Build history of the part. All positions in model axes, mm. A direction names the side the tool comes from. Round coordinates to 2 decimals unless told otherwise and drop trailing zeros. Write each loop counter-clockwise with the first axis right and the second up, starting at its lowest first coordinate (ties: lowest second). Pieces come first, ordered by that corner, then holes.
1) Pull direction X, two halves, no side cores. Call faces 6 (the flat face through (-145.011, 25, -16)), 7 (the cylindrical face through (-150.961, -14.765, -3.279)), 8 (the flat face through (-163.99, 16, -8)), 9 (the cylindrical face through (-146.66, -8.77, 27.84)): +X half, -X half, draft (parallel to the pull), parting line (faces both ways), or undercut.
2) Saw through at A-A (x = -81.5). Write the cut outline in (y, z), plus the area to 3 significant figures.
3) Which spindle directions (+Z, -Z, +X, -X, +Y, -Y) get a long thin tool onto all of the face, cutting with end or side? Do faces 1 (the flat face through (-90, -11.867, 0)), 2 (the conical face through (-144.014, -12.426, 39.459)), 3 (the flat face through (-122.028, 38, 92)), 4 (the cylindrical face through (-163.5, -4.84, 15.38)), 5 (the flat face through (-43.19, 7, 7)). Say none if no direction does.
4) Wall check: probe 1 along Y at (x, z) = (-163.45, 0) (3 decimals); probe 2 along Y at (x, z) = (-148, 0) (3 decimals); probe 3 along X at (y, z) = (57.5, -5). Give the ranges that are in metal, low to high.
5) Flat gauge pins, fed straight in: pin 1 (12 mm diameter, centred on x = -113, z = -47, fed in from -Y); pin 2 (2.5 mm diameter, centred on x = -74.5, z = -1, fed in from +Y); pin 3 (1.5 mm diameter, centred on x = -72.5, z = -21.5, fed in from +Y); pin 4 (24 mm diameter, centred on y = 0, z = 0, fed in from +X). Where does each tip first touch, or does it go through?
from build123d import *

# Parameters (mm, degrees)
SKETCH2_R          = 15.125
CUT_EXTRUDE5_DEPTH = 24.4
CUT_EXTRUDE6_REACH = 177.309
SKETCH3_R          = 9.543
CUT_EXTRUDE7_REACH = 192.328
SKETCH4_W          = 4.8
SKETCH4_H          = 4.648


with BuildPart() as part:
    # Sketch1 → Revolve1 (revolve)
    with BuildSketch(Plane.XY, mode=Mode.PRIVATE) as revolve1_sk:
        Polygon((-162.990125159, 0), (-162.990125159, 16.125), (-163.990125159, 16.125), (-163.990125159, 37.741454009), (-160.123125159, 37.741454009), (-160.123125159, 99), (-159.313606376, 99), (-159.313606376, 104), (-159.063606376, 104), (-159.063606376, 99), (-148.352353258, 37.189964302), (-148.352353258, 29.189964302), (-145.01123533, 29.189964302), (-145.01123533, 37.189964302), (-129.063606376, 104), (-122.028125159, 104), (-122.028125159, 99), (-89.190125159, 99), (-89.190125159, 55), (-49.716595762, 55), (-44.190125159, 29), (-44.190125159, 16.015195652), (-43.190125159, 16.015195652), (-43.190125159, 0), align=None)
    revolve(revolve1_sk.sketch.rotate(Axis((-162.990125159, 0, 0), (1, 0, 0)), 90), axis=Axis((-162.990125159, 0, 0), (1, 0, 0)))

    # Sketch2 → Cut-Extrude5 (cut)
    with BuildSketch(Plane.ZY.offset(162.990125159)):
        Circle(SKETCH2_R)
    extrude(amount=-CUT_EXTRUDE5_DEPTH, mode=Mode.SUBTRACT)

    # Sketch3 → Cut-Extrude6 (cut, up to next)
    with BuildSketch(Plane.ZY.offset(138.590125159), mode=Mode.PRIVATE) as cut_extrude6_sk1:
        Circle(SKETCH3_R)
    cut_extrude6_tool1 = extrude(cut_extrude6_sk1.sketch, amount=-CUT_EXTRUDE6_REACH, mode=Mode.PRIVATE) & part.part
    add(cut_extrude6_tool1.solids().sort_by_distance((-138.590125, 0, 0))[0], mode=Mode.SUBTRACT)

    # Sketch4 → Cut-Extrude7 (cut, up to next)
    with BuildSketch(Plane(origin=(-43.190125159, 0, 0), x_dir=(0, 0, -1), z_dir=(1, 0, 0)), mode=Mode.PRIVATE) as cut_extrude7_sk1:
        with Locations((0, -9.543)):
            Rectangle(SKETCH4_W, SKETCH4_H)
    cut_extrude7_tool1 = extrude(cut_extrude7_sk1.sketch, amount=-CUT_EXTRUDE7_REACH, mode=Mode.PRIVATE) & part.part
    add(cut_extrude7_tool1.solids().sort_by_distance((-43.190125, -9.543, 0))[0], mode=Mode.SUBTRACT)


solid = part.part
Evaluation:
1. face 6: undercut
1. face 7: draft
1. face 8: -X half
1. face 9: undercut
2. outline: circle Ø110 at (0, 0); hole (-11.87, -2.4) - (-9.24, -2.4) arc R9.54 ccw (long way) to (-9.24, 2.4) - (-11.87, 2.4) - close
2. area: 9,210 mm2
3. face 1: +X, -X
3. face 2: none
3. face 3: +X
3. face 4: -X
3. face 5: +Z, -Z, +X, +Y, -Y
4. probe 1: y = -37.741 to -16.125, 16.125 to 37.741
4. probe 2: y = -29.19 to -15.125, 15.125 to 29.19
4. probe 3: x = -160.12 to -151.91, -140.11 to -89.19
5. pin 1: stops at y = -90.11
5. pin 2: stops at y = 55
5. pin 3: stops at y = 50.94
5. pin 4: stops at x = -43.19
